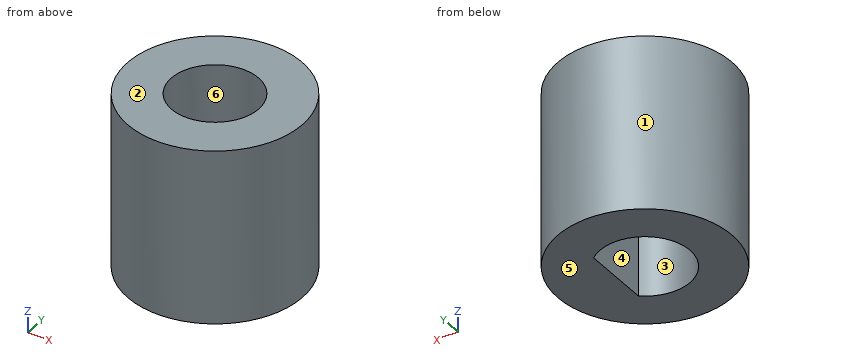
from build123d import *

# Parameters (mm, degrees)
BOSS_EXTRUDE1_START = 15
SKETCH1_R           = 6
BOSS_EXTRUDE1_DEPTH = 12
CUT_EXTRUDE2_DEPTH  = 6
SKETCH2_R           = 3
CUT_EXTRUDE1_DEPTH  = 6


with BuildPart() as part:
    # Sketch1 → Boss-Extrude1 (new body)
    with BuildSketch(Plane.XY.offset(BOSS_EXTRUDE1_START)):
        with Locations((16.35, -29.65)):
            Circle(SKETCH1_R)
    extrude(amount=BOSS_EXTRUDE1_DEPTH)

    # Sketch3 → Cut-Extrude2 (cut)
    with BuildSketch(Plane(origin=(0, 0, 15), x_dir=(-1, 0, 0), z_dir=(0, 0, -1))):
        with BuildLine():
            Line((-18.35, -32.018543856), (-18.35, -27.281456144))
            ThreePointArc((-18.35, -27.281456144), (-13.25, -29.65), (-18.35, -32.018543856))
        make_face()
    extrude(amount=-CUT_EXTRUDE2_DEPTH, mode=Mode.SUBTRACT)

    # Sketch2 → Cut-Extrude1 (cut)
    with BuildSketch(Plane.XY.offset(27)):
        with Locations((16.35, -29.65)):
            Circle(SKETCH2_R)
    extrude(amount=-CUT_EXTRUDE1_DEPTH, mode=Mode.SUBTRACT)


solid = part.part
Build history of the part. All positions in model axes, mm. Face numbers are marked on the shaded views. A direction names the side the tool comes from. Coordinates: 2 decimals unless noted, no trailing zeros. Write each loop counter-clockwise with the first axis right and the second up, starting at its lowest first coordinate (ties: lowest second). Pieces come first, ordered by that corner, then holes.
(1) Cut at D-D on y = -33.25. List the corners of the cut face in (x, z).
(2) Cut at C-C on z = 24.5. List the corners of the cut face in (x, y), and give its area (3 significant figures).
(3) Cut at B-B on x = 16.35. List the corners of the cut face in (y, z), and give its area (3 significant figures).
(4) Cut at A-A on y = -29.65. List the corners of the cut face in (x, z), and give its area (3 significant figures).
(5) Drill centre lines: line 1 (Y direction, x = 16.35, z = 24.75); line 2 (Y direction, x = 16.35, z = 19.7); line 3 (X direction, y = -27, z = 23.5). Where is each one in solid material? Low to high.
(6) 3-axis set-ups, long thin cutter, end or side, ignore diameter. For the marked faces 5 and 6: which of +Z, -Z, +X, -X, +Y, -Y reach the whole face in a straight line?
(7) Pin check, flat tips, straight feed: pin 1 Ø7 at (x, y) = (16.35, -29.65) entering from +Z; pin 2 Ø2 at (y, z) = (-32, 21.5) entering from +X; pin 3 Ø1.5 at (x, y) = (15, -30.5) entering from +Z; pin 4 Ø5 at (x, z) = (12.5, 25) entering from -Y. Stop position of each tip, or through.
(8) Mould opens along Y. For the marked faces 1, 2, 3 and 4 say: pulls with the +Y half, pulls with the -Y half, needs draft (parallel to the pull), parting line crosses it, or undercut.
Working result:
1. outline: (11.55, 15) - (21.15, 15) - (21.15, 27) - (11.55, 27) - close
2. outline: circle Ø12 at (16.35, -29.65); hole circle Ø6 at (16.35, -29.65)
2. area: 84.8 mm2
3. outline: (-35.65, 15) - (-32.75, 15) - (-32.75, 21) - (-32.65, 21) - (-32.65, 27) - (-35.65, 27) - close; (-26.65, 21) - (-26.55, 21) - (-26.55, 15) - (-23.65, 15) - (-23.65, 27) - (-26.65, 27) - close
3. area: 70.8 mm2
4. outline: (10.35, 15) - (13.25, 15) - (13.25, 21) - (13.35, 21) - (13.35, 27) - (10.35, 27) - close; (18.35, 15) - (22.35, 15) - (22.35, 27) - (19.35, 27) - (19.35, 21) - (18.35, 21) - close
4. area: 77.4 mm2
5. line 1: y = -35.65 to -32.65, -26.65 to -23.65
5. line 2: y = -35.65 to -32.75, -26.55 to -23.65
5. line 3: x = 10.97 to 14.94, 17.76 to 21.73
6. face 5: -Z, +X, -X, +Y, -Y
6. face 6: +Z
7. pin 1: stops at z = 27
7. pin 2: stops at x = 22.2
7. pin 3: passes through
7. pin 4: stops at y = -35.5
8. face 1: parting line crosses it
8. face 2: needs draft
8. face 3: undercut
8. face 4: undercut
